Model file for the job. Use its own axes, mm. A direction names the side the tool comes from. Round coordinates to 2 decimals unless told otherwise and drop trailing zeros. Order: outer loops, then holes, each group sorted by start corner. A loop starts at its lowest first (then second) coordinate and runs counter-clockwise, first axis right, second up. Notation, with made-up numbers: M 74,32.5 L 119,32.5 A7 ccw 119,38.5 Z; hole C 10.5,28 d5. An arc over 180 degrees is marked long. Return JSON: item names as keys, results as strings. Group by question number.
Item 1: Pin check, flat tip, straight feed: pin 1 Ø5 at (x, z) = (-2.5, 20) entering from +Y. Stop position of the tip, or through.
Item 2: Slice it at B-B on y = -0.5. Write the cut outline in (x, z) (3 decimals).
Item 3: Which spindle directions (+Z, -Z, +X, -X, +Y, -Y) get a long thin tool onto all of the face, cutting with end or side? Do faces 1 (the face through (1.798, 18.957, 6.107)), 2 (the face through (2, 0, 25.4)), 3 (the face through (0, -3.81, 13)). Say none if no direction does.
Item 4: Probe line 1 along Z through (x, y) = (-1, 1); line 2 along Y through (x, z) = (-2, 17.5); line 3 along Y through (x, z) = (0, 3.25). List the from-to ranges inside material, lowest first.
Item 5: Pull direction Z, two halves, no side cores. Call faces 4 (the face through (1.521, -11.79, 24.445)), 5 (the face through (1.8, 19, 19.5)), 6 (the face through (4, 25.396, 6)), 7 (the face through (2, 0, 0)): pulls with the +Z half, pulls with the -Z half, needs draft (parallel to the pull), parting line crosses it, or undercut.
Autodesk Inventor part; units mm, degrees
ref_plane "YZ Plane" through (0, 0, 0) normal (1, 0, 0) x (0, 1, 0)
ref_plane "XZ Plane" through (0, 0, 0) normal (0, 1, 0) x (-1, 0, 0)
ref_plane "XY Plane" through (0, 0, 0) normal (0, 0, 1) x (1, 0, 0)
sketch "Sketch1" plane through (0, 0, 0) normal (0, 0, 1) x (1, 0, 0)
  line L0 (6.35, -12.6955) -> (-3.175, -12.6955)
  line L1 (-6.35, -9.5205) -> (-6.35, 9.5205)
  line L2 (-3.175, 12.6955) -> (6.35, 12.6955)
  line L3 (6.35, 12.6955) -> (6.35, -12.6955)
  line L4 (6.35, -12.6955) -> (-6.35, 12.6955) construction
  line L5 (-6.35, -12.6955) -> (6.35, 12.6955) construction
  arc A0 (-3.175, 12.6955) -> (-6.35, 9.5205) centre (-3.175, 9.5205) ccw
  arc A1 (-6.35, -9.5205) -> (-3.175, -12.6955) centre (-3.175, -9.5205) ccw
  point P0 (0, 0)
  dimension "d0" = 12.7
  dimension "d1" = 3.175
extrude "Extrusion1" add sketch "Sketch1" along normal blind 25.4
fillet "Fillet1" radius 3.175 10 edges at (-6.35, 0, 25.4) (-5.4201, -11.7656, 25.4) (1.5875, -12.6955, 25.4) (1.5875, 12.6955, 25.4) (-5.4201, 11.7656, 25.4) (-5.4201, 11.7656, 0) (1.5875, 12.6955, 0) (-5.4201, -11.7656, 0) (1.5875, -12.6955, 0) (-6.35, 0, 0)
sketch "Sketch2" plane through (-3.175, 12.6955, 3.175) normal (0, 1, 0) x (1, 0, 0)
  arc A0 (9.525, -14.6582) -> (9.525, -17.7537) centre (7.511, -16.206) ccw
  line L0 (0, 0) -> (0, -19.05)
  line L1 (9.525, 0) -> (9.525, -19.05)
  arc A1 (9.525, -1.2963) -> (9.525, -4.3918) centre (7.511, -2.844) ccw
  line L2 (9.525, -1.2963) -> (9.525, -4.3918)
  line L3 (9.525, -14.6582) -> (9.525, -17.7537)
  point P0 (3.175, 3.175)
  dimension "d5" = 5.08
extrude "Extrusion2" add sketch "Sketch2" along normal blind 12.7
sketch "Sketch3" plane through (-6.35, -9.5205, 3.175) normal (-1, 0, 0) x (0, 0, 1)
  line L0 (4.445, 6.9805) -> (9.525, 9.5205) construction
  line L1 (9.525, 9.5205) -> (4.445, 11.5525) construction
  line L2 (3.175, 6.9805) -> (9.525, 9.5205) construction
  line L3 (9.525, 9.5205) -> (5.2917, 12.0605) construction
  line L4 (5.2917, 6.9805) -> (13.7583, 12.0605) construction
  line L5 (3.175, 13.3305) -> (3.175, 5.7105)
  line L6 (15.875, 5.7105) -> (15.875, 13.3305)
  line L7 (14.9679, 13.3305) -> (3.175, 5.0755) construction
  line L8 (4.0821, 13.3305) -> (14.9679, 5.7105) construction
  line L9 (3.175, 5.0755) -> (3.175, 5.7105)
  line L10 (15.875, 5.7105) -> (15.875, 13.3305)
  line L11 (3.175, 13.3305) -> (3.175, 5.7105)
  line L12 (3.175, 13.3305) -> (15.875, 13.3305)
  line L13 (3.175, 5.7105) -> (15.875, 5.7105)
  point P0 (-3.175, 9.5205)
  point P1 (9.525, 9.5205)
extrude "Extrusion3" cut sketch "Sketch3" against normal blind 12.7
properties part number "pig_butt"
Output values:
{
 "1": {"pin 1": "y = 12.7"},
 "2": {"outline": "M -6.35,3.175 A3.175 ccw -3.175,0 L 6.35,0 L 6.35,6.35 L -6.35,6.35 Z; M -6.35,19.05 L 6.35,19.05 L 6.35,25.4 L -3.175,25.4 A3.175 ccw -6.35,22.225 Z"},
 "3": {"face 1": "+Y", "face 2": "+Z, +X, -X, +Y, -Y", "face 3": "+X, -X"},
 "4": {"line 1": "0 to 6.35, 19.05 to 25.4", "line 2": "-12.7 to -3.81, 3.81 to 12.7", "line 3": "-12.7 to 12.7"},
 "5": {"face 4": "pulls with the +Z half", "face 5": "undercut", "face 6": "needs draft", "face 7": "pulls with the -Z half"}
}
